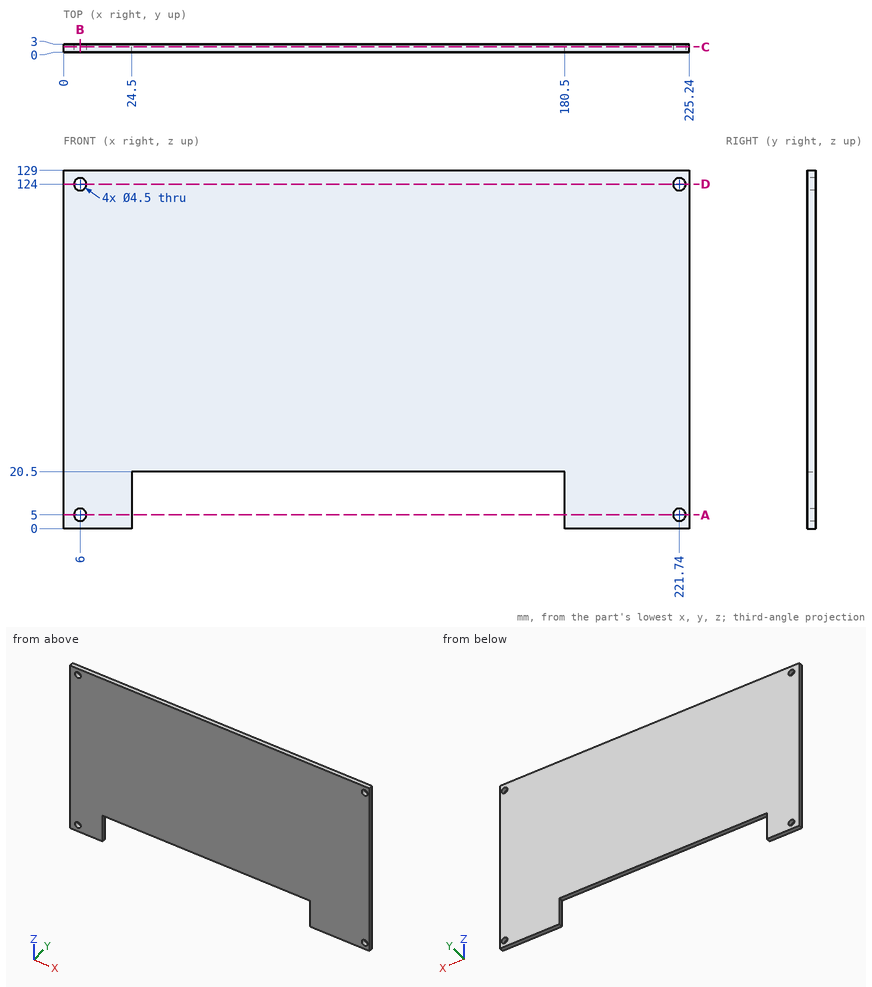
Job drawing, mm, ordinate dimensions from the low corner. One solid piece. Round coordinates to 2 decimals unless told otherwise and drop trailing zeros. Loops run counter-clockwise (first coordinate to the right, second up) from the corner with the lowest first, then second, coordinate; pieces in that order, holes last. Notation, with made-up numbers: (74.25, 59.5) -> (89.25, 59.5) arc R5 cw to (89.25, 64.5) -> close; hole circle Ø11 at (43.25, 41.5). An arc over 180 degrees is marked (long way). Use CSV: the item, a comma, the result in double quotes. Start each with the question number.
Q1. Flat gauge pin, fed straight in: pin 1 Ø1 at (x, y) = (127.5, 1) entering from -Z. Where does the tip first touch, or does it go through?
Q2. Saw through at D-D on z = 124. Give the cut face in (x, y), and give its area (3 significant figures).
Q3. Saw through at A-A on z = 5. Give the cut face in (x, y).
Q4. Saw through at C-C on y = 1.95. Give the cut face in (x, z), and give its area (3 significant figures).
Q5. Drill centre lines: L1, parallel to Z at x = 6, y = 1.95; L2, parallel to X at y = 2.3, z = 5; L3, parallel to X at y = 0.7, z = 124. Where is each one in solid material? Low to high.
Q6. Saw through at B-B on x = 6. Give the cut face in (y, z).
Solutions:
1,pin 1,"stops at z = 20.5"
2,outline,"(0, 0) -> (3.75, 0) -> (3.75, 3) -> (0, 3) -> close; (8.25, 0) -> (219.49, 0) -> (219.49, 3) -> (8.25, 3) -> close; (223.99, 0) -> (225.24, 0) -> (225.24, 3) -> (223.99, 3) -> close"
2,area,"649 mm^2"
3,outline,"(0, 0) -> (3.75, 0) -> (3.75, 3) -> (0, 3) -> close; (8.25, 0) -> (24.5, 0) -> (24.5, 3) -> (8.25, 3) -> close; (180.5, 0) -> (219.49, 0) -> (219.49, 3) -> (180.5, 3) -> close; (223.99, 0) -> (225.24, 0) -> (225.24, 3) -> (223.99, 3) -> close"
4,outline,"(0, 0) -> (24.5, 0) -> (24.5, 20.5) -> (180.5, 20.5) -> (180.5, 0) -> (225.24, 0) -> (225.24, 129) -> (0, 129) -> close; hole circle Ø4.5 at (6, 5); hole circle Ø4.5 at (6, 124); hole circle Ø4.5 at (221.74, 5); hole circle Ø4.5 at (221.74, 124)"
4,area,"25,800 mm^2"
5,L1,"z = 0 to 2.75, 7.25 to 121.75, 126.25 to 129"
5,L2,"x = 0 to 3.75, 8.25 to 24.5, 180.5 to 219.49, 223.99 to 225.24"
5,L3,"x = 0 to 3.75, 8.25 to 219.49, 223.99 to 225.24"
6,outline,"(0, 0) -> (3, 0) -> (3, 2.75) -> (0, 2.75) -> close; (0, 7.25) -> (3, 7.25) -> (3, 121.75) -> (0, 121.75) -> close; (0, 126.25) -> (3, 126.25) -> (3, 129) -> (0, 129) -> close"
